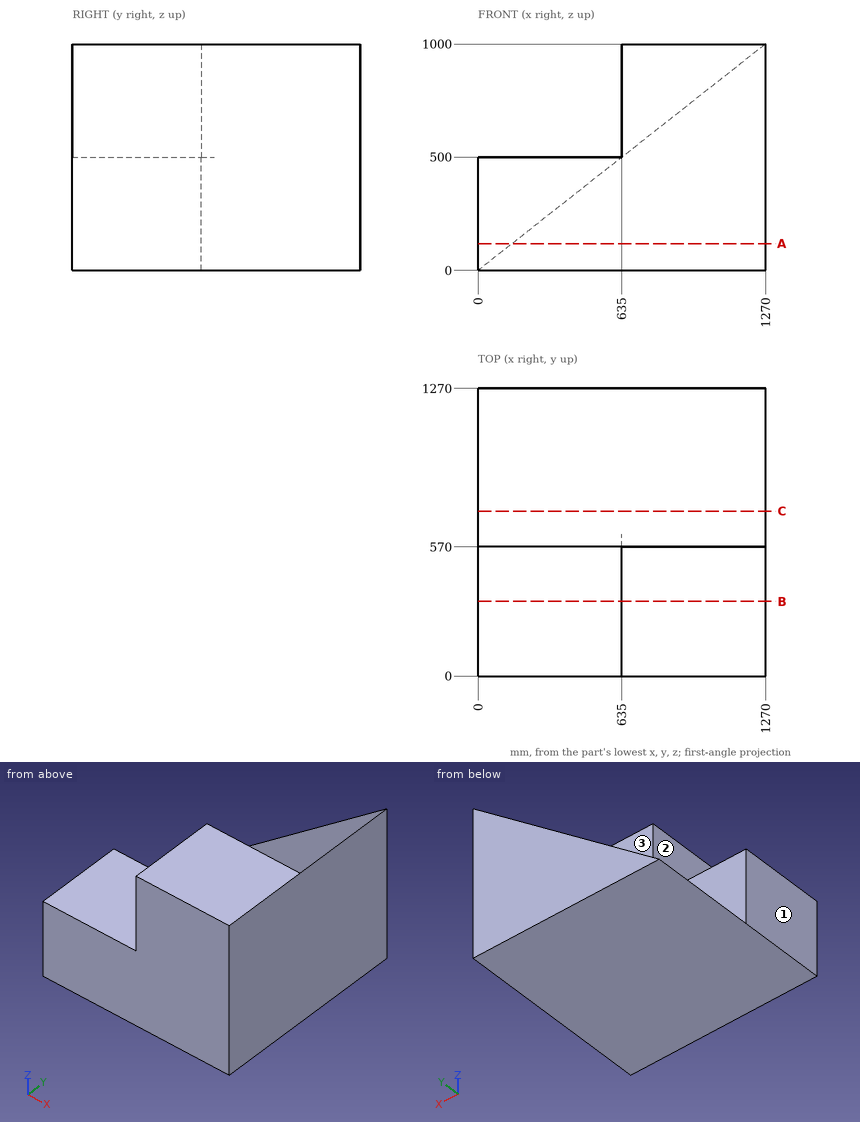
Could you check a few things on this drawing? It's one solid part, dimensions in mm from its lowest x, y, z. A direction names the side the tool comes from. Give positions to 0.01 mm unless a question says otherwise; leave off trailing zeros. Write each loop counter-clockwise with the first axis right and the second up, starting at its lowest first coordinate (ties: lowest second). Pieces come first, ordered by that corner, then holes. Notation, with made-up numbers: (-1.5, -23) -> (49.5, -23) arc R8 ccw to (49.5, -18) -> close; hole circle Ø3 at (50.5, 72). An arc over 180 degrees is marked (long way). Answer as CSV lines item,"result". Start each with the question number.
(1) If we section it at A-A, the plane z = 118: Write out the boundary of the cut face in (x, y).
(2) If we section it at B-B, the plane y = 329.5: Write out the boundary of the cut face in (x, z), and give its area (4 significant figures).
(3) I'm going to push flat-ended pins straight in: pin 1 Ø5 at (y, z) = (1122, 268.5) entering from -X; pin 2 Ø12 at (x, y) = (1021.5, 1091.5) entering from +Z; pin 3 Ø5 at (y, z) = (500, 816) entering from -X. Where does each tip first touch, or does it pass through?
(4) Please list where these lines run through material, in increasing order: line 1 (Y direction, x = 342.5, z = 330.5); line 2 (Z direction, x = 520, y = 513.5); line 3 (X direction, y = 333.5, z = 931).
(5) If we section it at C-C, the plane y = 728: Write out the boundary of the cut face in (x, z).
(6) Which directions (+Z, -Z, +X, -X, +Y, -Y) give clear straight access to the entire face, cutting with the end or side of a thin tool? Please do the marked faces 1, 2 and 3.
Answer list:
1,outline,"(0, 0) -> (1270, 0) -> (1270, 1270) -> (149.86, 1270) -> (149.86, 570) -> (0, 570) -> close"
2,outline,"(0, 0) -> (1270, 0) -> (1270, 1000) -> (635, 1000) -> (635, 500) -> (0, 500) -> close"
2,area,"952,500 mm^2"
3,pin 1,"x = 337.82"
3,pin 2,"z = 809.06"
3,pin 3,"x = 635"
4,line 1,"0 to 570"
4,line 2,"0 to 500"
4,line 3,"635 to 1270"
5,outline,"(0, 0) -> (1270, 0) -> (1270, 1000) -> close"
6,face 1,"+Z, -Z, -X, +Y, -Y"
6,face 2,"+Z, -X, +Y, -Y"
6,face 3,"+Z, -X, +Y"
